Here's how the part is built. I have some questions about the finished solid (model axes, mm). Coordinates: 2 decimals unless noted, no trailing zeros. Write each loop counter-clockwise with the first axis right and the second up, starting at its lowest first coordinate (ties: lowest second). Pieces come first, ordered by that corner, then holes.
```python
from build123d import *

# Parameters (mm, degrees)
BOSS_EXTRUDE1_DEPTH     = 19.05
CUT_EXTRUDE1_DEPTH      = 295.751251025
CUT_EXTRUDE1_DEPTH_BACK = 295.751251025
SKETCH2_W               = 12.7
SKETCH2_H               = 12.7


with BuildPart() as part:
    # Sketch1 → Boss-Extrude1 (new body)
    with BuildSketch(Plane(origin=(0, 0, 0), x_dir=(0, 0, -1), z_dir=(1, 0, 0))):
        Polygon((249.444858146, -198.74145037), (268.494858146, -191.807817407), (94.609985754, 15.420103965), (88.9, 22.225), (81.966367037, 3.175), align=None)
    extrude(amount=BOSS_EXTRUDE1_DEPTH)

    # Sketch2 → Cut-Extrude1 (cut, two sides: drawn at the far end of the back side and taken through both)
    with BuildSketch(Plane(origin=(0, -244.765356655, -205.382520494), x_dir=(-1, 0, 0), z_dir=(0, -0.766044443118953, -0.6427876096865692)).offset(-CUT_EXTRUDE1_DEPTH_BACK)):
        with Locations((-9.525, 72.862305619)):
            Rectangle(SKETCH2_W, SKETCH2_H)
    extrude(amount=CUT_EXTRUDE1_DEPTH + CUT_EXTRUDE1_DEPTH_BACK, mode=Mode.SUBTRACT)


solid = part.part
```
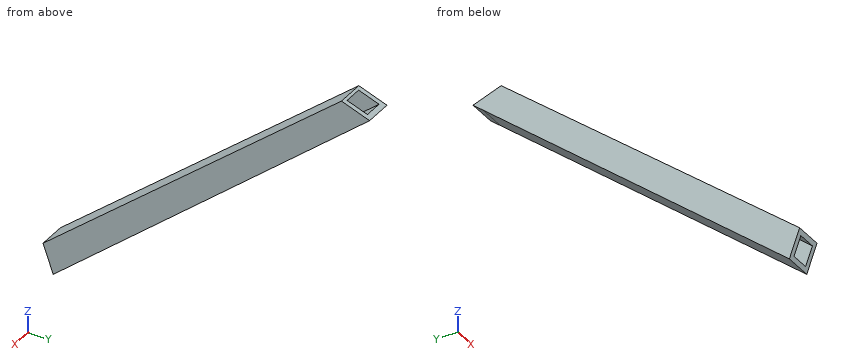
1) Will these pins go through, and if not, where does the flat tip stop? pin 1 (6 mm diameter, centred on x = 15, z = -187, fed in from +Y); pin 2 (5 mm diameter, centred on x = 16, z = -106.5, fed in from +Y); pin 3 (1 mm diameter, centred on x = 4.5, y = -172, fed in from +Z).
Values follow:
pin 1: stops at y = -91.11
pin 2: stops at y = 4.23
pin 3: stops at z = -226.85
2) Imagine slicing it at A-A on x = 9. Please give me the cut outline in (y, z) (3 decimals), then the cut area to 3 significant figures.
Values follow:
outline: (-198.741, -249.445) - (-197.586, -252.62) - (5, -82.63) - (3.175, -81.966) - close; (-192.963, -265.32) - (-191.808, -268.495) - (22.225, -88.9) - (18.78, -87.646) - close
area: 1,520 mm2
3) Imagine slicing it at B-B on y = -81. Please give me the cut outline in (x, z) (3 decimals), then the cut area to 3 significant figures.
Values follow:
outline: (0, -175.516) - (19.05, -175.516) - (19.05, -151.785) - (0, -151.785) - close; hole (3.175, -171.371) - (15.875, -171.371) - (15.875, -154.793) - (3.175, -154.793) - close
area: 242 mm2
4) Imagine slicing it at C-C on z = -113.5. Please give me the cut outline in (x, y) (3 decimals).
Values follow:
outline: (0, -34.843) - (19.05, -34.843) - (19.05, -7.092) - (0, -7.092) - close; hole (3.175, -31.789) - (15.875, -31.789) - (15.875, -12.032) - (3.175, -12.032) - close
5) I need wall thicknesses on probe 1 along X at (y, z) = (-130, -201) (3 decimals); probe 2 along Y at (x, z) = (7.5, -190); probe 3 along Y at (x, z) = (7.5, -166). Which ranges of each line are inside material? Lowest first, please.
Values follow:
probe 1: x = 0 to 3.175, 15.875 to 19.05
probe 2: y = -127.07 to -122.96, -103.2 to -98.26
probe 3: y = -98.14 to -94.36, -74.6 to -69.66
